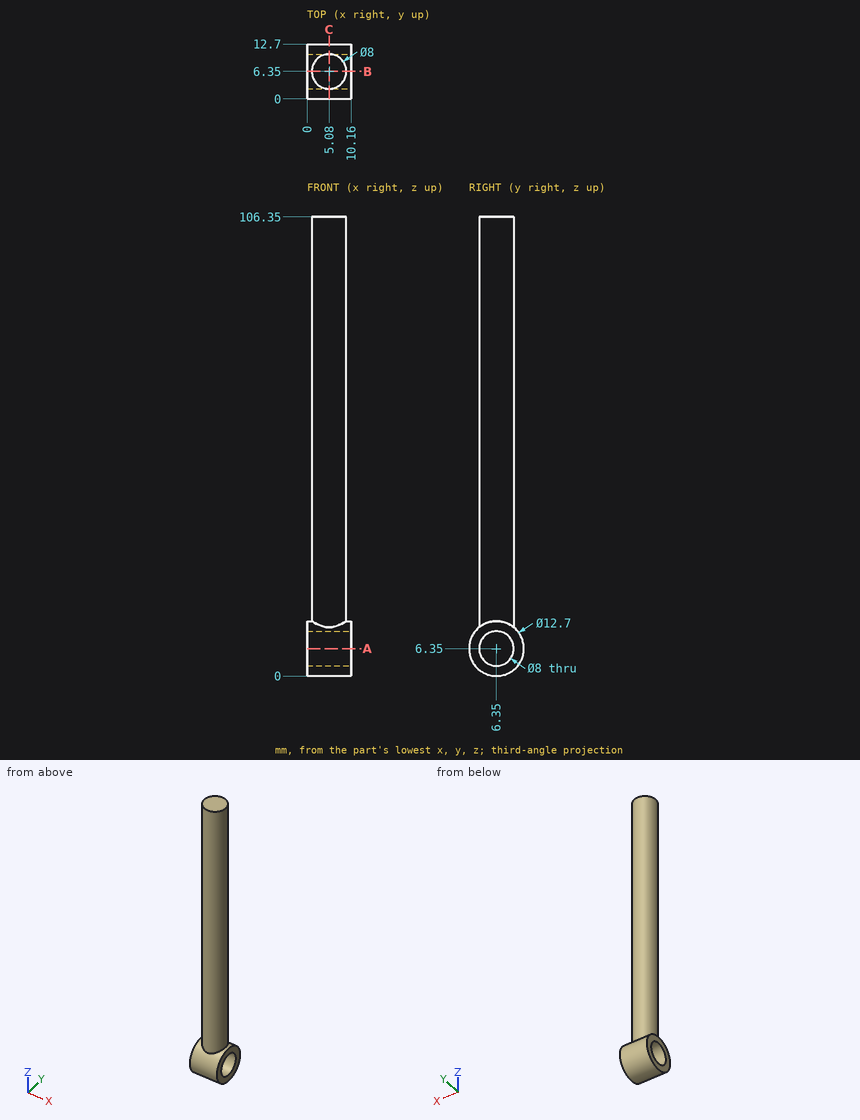
Study the drawing (mm; zero at the part's minimum x, y, z) and answer. Coordinates: 2 decimals unless noted, no trailing zeros. Write each loop counter-clockwise with the first axis right and the second up, starting at its lowest first coordinate (ties: lowest second). Pieces come first, ordered by that corner, then holes.
Q1. Given P1, Ø3, axis at x = 4, z = 29, coming from the -Y side; P2, Ø6, axis at y = 5.5, z = 60.5, coming from the -X side; P3, Ø6, axis at x = 7, z = 66, coming from the +Y side, each flat-ended and moving along its own axis, determine where each tip first touches the part or whether it passes through.
Returned:
P1: stops at y = 2.35
P2: stops at x = 1.08
P3: stops at y = 10.35
Q2. Section B-B, the plane y = 6.35 is taken. Write down the section's boundary in (x, z).
Returned:
outline: (0, 0) - (10.16, 0) - (10.16, 2.35) - (0, 2.35) - close; (0, 10.35) - (10.16, 10.35) - (10.16, 12.7) - (9.08, 12.7) - (9.08, 106.35) - (1.08, 106.35) - (1.08, 12.7) - (0, 12.7) - close
Q3. Section C-C, the plane x = 5.08 is taken. Write down the section's boundary in (y, z).
Returned:
outline: (2.35, 11.28) arc R6.35 ccw (long way) to (10.35, 11.28) - (10.35, 106.35) - (2.35, 106.35) - close; hole circle Ø8 at (6.35, 6.35)
Q4. Find the intervals of material crossed by line 1 along Y through (x, z) = (5.75, 6.35); line 2 along X through (y, z) = (6.75, 71.5); line 3 along Z through (x, y) = (6.5, 7), in increasing order.
Returned:
line 1: y = 0 to 2.35, 10.35 to 12.7
line 2: x = 1.1 to 9.06
line 3: z = 0.03 to 2.4, 10.3 to 106.35
Q5. Section A-A, the plane z = 6.35 is taken. Write down the section's boundary in (x, y).
Returned:
outline: (0, 0) - (10.16, 0) - (10.16, 2.35) - (0, 2.35) - close; (0, 10.35) - (10.16, 10.35) - (10.16, 12.7) - (0, 12.7) - close
